For this review, use the dimensioned drawing (mm, ordinates from the lowest corner) and the shaded views. Round coordinates to 2 decimals unless told otherwise and drop trailing zeros. Write each loop counter-clockwise with the first axis right and the second up, starting at its lowest first coordinate (ties: lowest second). Pieces come first, ordered by that corner, then holes.
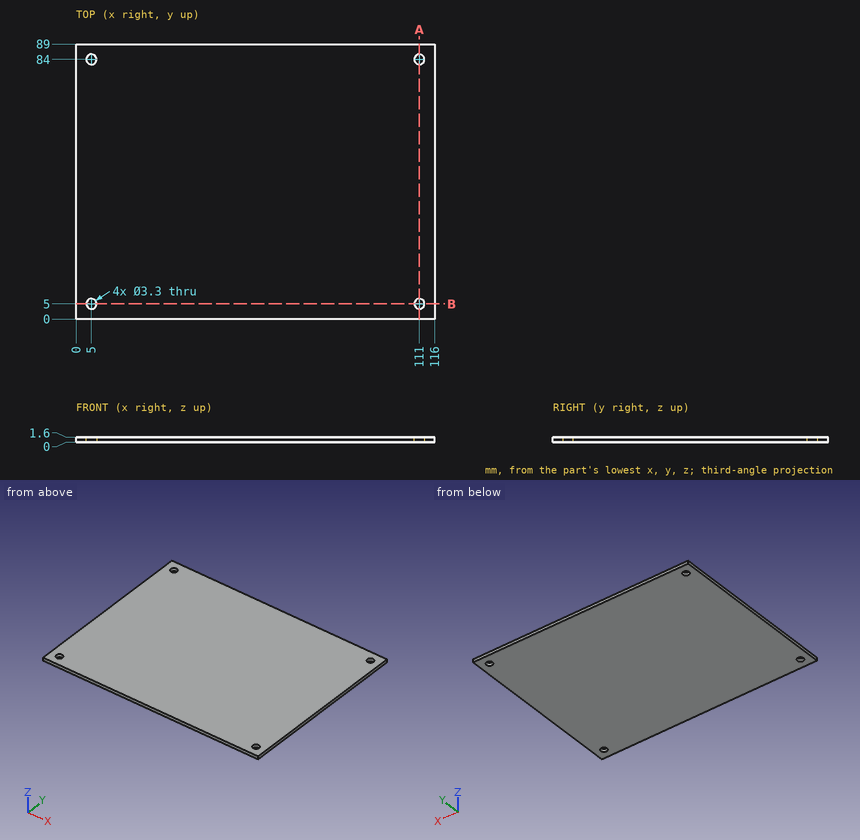
1) For line 1 along Y through (x, z) = (111, 0.8); line 2 along X through (y, z) = (84, 1.15); line 3 along Y through (x, z) = (6, 1.1), list the stretches that pass through material, from the lowest coordinate up.
2) For P1, Ø3, axis at x = 111, y = 84, coming from the +Z side, flat-tipped, find the tip position at first contact; note if it passes through.
3) Add section B-B on y = 5. State the section outline as (x, z) points, and give its area (3 significant figures).
4) Add section A-A on x = 111. State the section outline as (y, z) points.
Computed:
1. line 1: y = 0 to 3.35, 6.65 to 82.35, 85.65 to 89
1. line 2: x = 0 to 3.35, 6.65 to 109.35, 112.65 to 116
1. line 3: y = 0 to 3.69, 6.31 to 82.69, 85.31 to 89
2. P1: passes through
3. outline: (0, 0) - (3.35, 0) - (3.35, 1.6) - (0, 1.6) - close; (6.65, 0) - (109.35, 0) - (109.35, 1.6) - (6.65, 1.6) - close; (112.65, 0) - (116, 0) - (116, 1.6) - (112.65, 1.6) - close
3. area: 175 mm2
4. outline: (0, 0) - (3.35, 0) - (3.35, 1.6) - (0, 1.6) - close; (6.65, 0) - (82.35, 0) - (82.35, 1.6) - (6.65, 1.6) - close; (85.65, 0) - (89, 0) - (89, 1.6) - (85.65, 1.6) - close
